Source: three-view drawing plus pictorial views. Frame: mm from the lowest corner of the part. A direction names the side the tool comes from. Give positions to 0.01 mm unless a question says otherwise; leave off trailing zeros. Order: outer loops, then holes, each group sorted by start corner. A loop starts at its lowest first (then second) coordinate and runs counter-clockwise, first axis right, second up. Notation, with made-up numbers: (15.25, 60) - (22.25, 60) arc R21 cw to (22.25, 64) - close; hole circle Ø6 at (-23.75, 45). An arc over 180 degrees is marked (long way). Answer in a Markdown table with one row per item. Add a question column.
1. Section query B-B on z = 16. Return loops of the section in (x, y).
2. Section query A-A on y = 23.5. Return loops of the section in (x, z).
3. Contact query for flat-ended pins moving along their axis: pin 1 (5.5 mm diameter, centred on x = 11, z = 40, fed in from +Y) (1 decimal); pin 2 (18.5 mm diameter, centred on x = 17.5, y = 15.5, fed in from +Z). Output: stop coordinate, or through.
4. Ray query, line 1 (Y direction, x = 27, z = 7); line 2 (X direction, y = 1.5, z = 40); line 3 (Z direction, x = 25, y = 18). Return the intervals inside material, ascending. Write a range as [from, to].
5. Mould query, pull axis Y, two halves, no side actions, for the marked faces 3, 4, 5 and 6. Classes: released by +Y, released by -Y, zero draft, split by the parting line, or undercut.
6. Section query D-D on z = 41. Return loops of the section in (x, y).
7. Access query for the marked faces 1 and 2. Directions: +Z, -Z, +X, -X, +Y, -Y. A direction counts if a zero-diameter tool reaches every point of the face in a straight line with its end or side. Return the directions, or none.
8. Section query C-C on x = 11. Return loops of the section in (y, z).
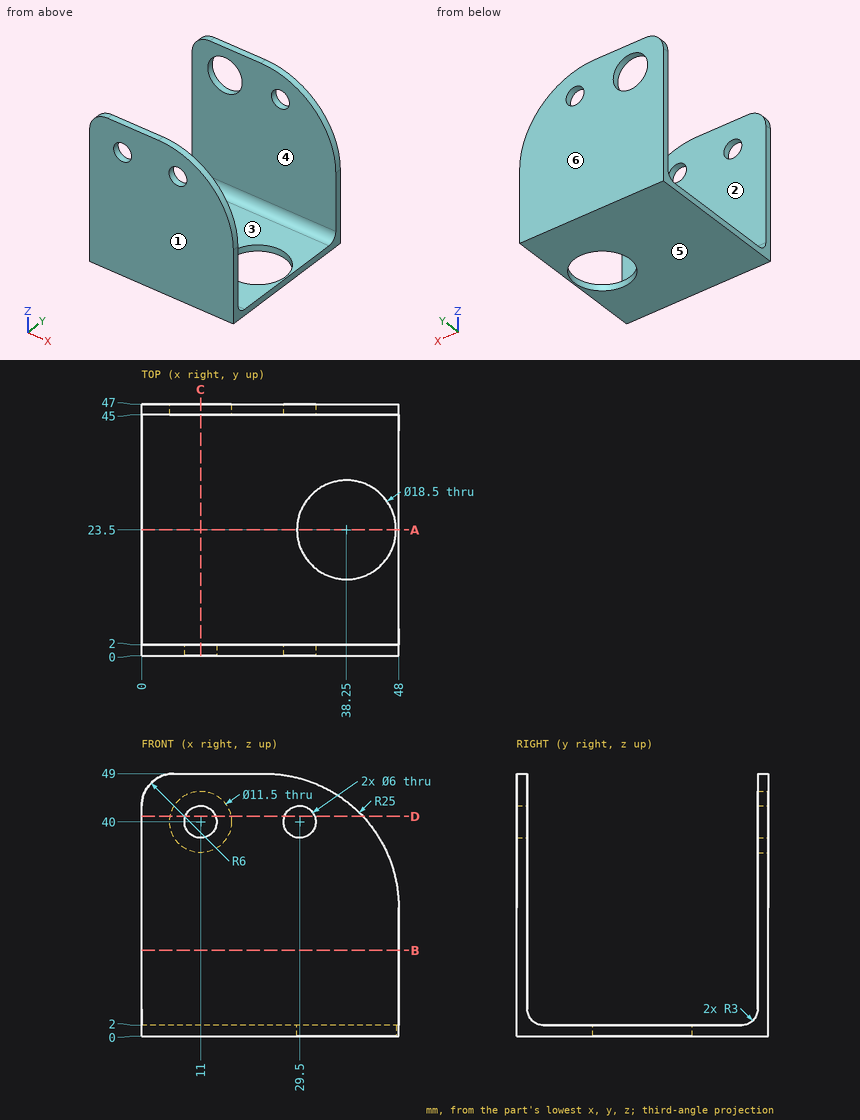
Answer:
| question | item | result |
|---|---|---|
| 1 | outline | (0, 0) - (48, 0) - (48, 2) - (0, 2) - close; (0, 45) - (48, 45) - (48, 47) - (0, 47) - close |
| 2 | outline | (0, 0) - (29, 0) - (29, 2) - (0, 2) - close; (47.5, 0) - (48, 0) - (48, 2) - (47.5, 2) - close |
| 3 | pin 1 | passes through |
| 3 | pin 2 | stops at z = 2 |
| 4 | line 1 | y = [0, 2], [45, 47] |
| 4 | line 2 | x = [0, 8], [14, 26.5], [32.5, 42.21] |
| 4 | line 3 | z = [0, 2] |
| 5 | face 3 | undercut |
| 5 | face 4 | undercut |
| 5 | face 5 | zero draft |
| 5 | face 6 | released by +Y |
| 6 | outline | (0, 0) - (8.17, 0) - (8.17, 2) - (0, 2) - close; (0, 45) - (5.34, 45) - (5.34, 47) - (0, 47) - close; (13.83, 0) - (26.67, 0) - (26.67, 2) - (13.83, 2) - close; (16.66, 45) - (26.67, 45) - (26.67, 47) - (16.66, 47) - close; (32.33, 0) - (41.33, 0) - (41.33, 2) - (32.33, 2) - close; (32.33, 45) - (41.33, 45) - (41.33, 47) - (32.33, 47) - close |
| 7 | face 1 | +Z, -Z, +X, -X, -Y |
| 7 | face 2 | +Z, +X, -X |
| 8 | outline | (0, 0) - (47, 0) - (47, 34.25) - (45, 34.25) - (45, 5) arc R3 cw to (42, 2) - (5, 2) arc R3 cw to (2, 5) - (2, 37) - (0, 37) - close; (0, 43) - (2, 43) - (2, 49) - (0, 49) - close; (45, 45.75) - (47, 45.75) - (47, 49) - (45, 49) - close |
